Design review of the part built by this model. Coordinates are the model's own, in mm. Face numbers are marked on the shaded views. A direction names the side the tool comes from. Coordinates: 2 decimals unless noted, no trailing zeros. Loops run counter-clockwise (first coordinate to the right, second up) from the corner with the lowest first, then second, coordinate; pieces in that order, holes last. Notation, with made-up numbers: M -33,-13.75 L 1,-13.75 A25 ccw 1,5.25 Z; hole C 66,21 d6. An arc over 180 degrees is marked long. Put each result on its own line as item: value. Start each with the question number.
(1) For probe 1 along Z at (x, y) = (25, -8.5); probe 2 along X at (y, z) = (-26, 50.5); probe 3 along Z at (x, y) = (5, -20.5), list the stretches that pass through material, from the lowest coordinate up. Write a range as [from, to].
(2) Take a section at C-C, the plane y = -27.5. Give the boundary of the cut face in (x, z).
(3) Take a section at D-D, the plane z = 55. Give the boundary of the cut face in (x, y), then the cut area to 3 significant figures.
(4) Clearance check with flat-ended pins moving along their axes: pin 1 (2 mm diameter, centred on y = -11, z = 16, fed in from -X); pin 2 (4 mm diameter, centred on y = -5, z = 16, fed in from -X); pin 3 (10 mm diameter, centred on y = -6, z = 40, fed in from +X). State where each tip first meets the part, or that it passes through.
(5) Take a section at B-B, the plane x = 25.4. Give the boundary of the cut face in (y, z).
(6) The part is to be moulded in two halves that separate along X. For the marked faces 6, 7 and 8, say which applies: +X half, -X half, draft (parallel to the pull), parting line (faces both ways), or undercut.
(7) Take a section at A-A, the plane y = -14. Give the boundary of the cut face in (x, z).
(8) For the marked faces 1, 2, 3, 4 and 5, list the 3-axis set-ups (+Z, -Z, +X, -X, +Y, -Y) from which the entire face can be reached by the end or side of a thin tool; tool diameter is ignored.
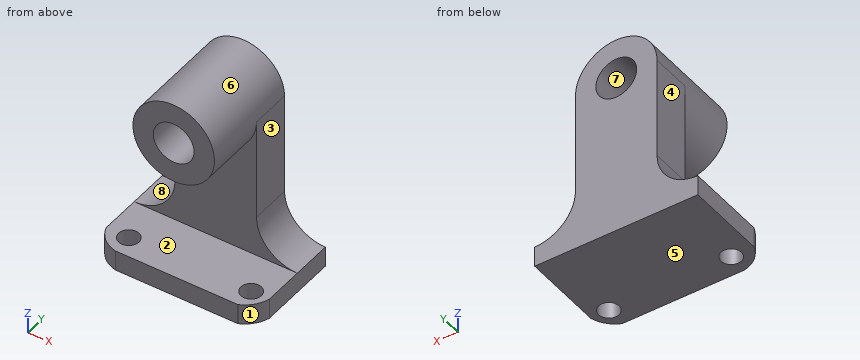
```python
from build123d import *

# Parameters (mm, degrees)
F1_DEPTH  = 31.75
F2_W      = 19.05
F2_H      = 31.75
F3_DEPTH  = 57.15
F5_DEPTH  = 19.05
F7_DEPTH  = 25.4
F8_R      = 6.35
F9_DEPTH  = 31.75
F11_DEPTH = 6.35
F12_R     = 3.175
F13_DEPTH = 6.35
F14_DEPTH = 6.35


with BuildPart() as f1:
    # F0 (on Front) → F1 (new body)
    with BuildSketch(Plane.XZ):
        Polygon((0, 6.35), (0, 0), (50.8, 0), (50.8, 6.35), (50.8, 63.5), (0, 63.5), align=None)
    extrude(amount=F1_DEPTH)

    # F2 (on face) → F3 (cut)
    with BuildSketch(Plane.YZ.offset(50.8)):
        with Locations((-22.225, 22.225)):
            Rectangle(F2_W, F2_H)
    extrude(amount=-F3_DEPTH, mode=Mode.SUBTRACT)

    # F4 (on face) → F5 (cut)
    with BuildSketch(Plane.XZ.offset(31.75)):
        with BuildLine():
            ThreePointArc((25.4, 63.5), (34.3802561211, 59.7802561211), (38.1, 50.8))
            ThreePointArc((38.1, 50.8), (34.3802561211, 41.8197438789), (25.4, 38.1))
            Line((25.4, 38.1), (50.8, 38.1))
            Line((50.8, 38.1), (50.8, 63.5))
            Line((50.8, 63.5), (25.4, 63.5))
        make_face()
        with BuildLine():
            ThreePointArc((25.4, 38.1), (12.7, 50.8), (25.4, 63.5))
            Line((25.4, 63.5), (0, 63.5))
            Line((0, 63.5), (0, 38.1))
            Line((0, 38.1), (25.4, 38.1))
        make_face()
    extrude(amount=-F5_DEPTH, mode=Mode.SUBTRACT)

    # F6 (on face) → F7 (cut)
    with BuildSketch(Plane.XZ.offset(12.7)):
        with BuildLine():
            Line((0, 63.5), (0, 6.35))
            ThreePointArc((0, 6.35), (8.9802561211, 10.0697438789), (12.7, 19.05))
            Line((12.7, 19.05), (12.7, 50.8))
            ThreePointArc((12.7, 50.8), (16.4197438789, 59.7802561211), (25.4, 63.5))
            Line((25.4, 63.5), (0, 63.5))
        make_face()
        with BuildLine():
            ThreePointArc((38.1, 19.05), (41.8197438789, 10.0697438789), (50.8, 6.35))
            Line((50.8, 6.35), (50.8, 63.5))
            Line((50.8, 63.5), (25.4, 63.5))
            ThreePointArc((25.4, 63.5), (34.3802561211, 59.7802561211), (38.1, 50.8))
            Line((38.1, 50.8), (38.1, 19.05))
        make_face()
    extrude(amount=-F7_DEPTH, mode=Mode.SUBTRACT)

    # F8 (on face) → F9 (cut)
    with BuildSketch(Plane.XZ.offset(31.75)):
        with Locations((25.4, 50.8)):
            Circle(F8_R)
    extrude(amount=-F9_DEPTH, mode=Mode.SUBTRACT)

    # F10 (on face) → F11 (cut)
    with BuildSketch(Plane.XY.offset(6.35)):
        with BuildLine():
            Line((0, -25.4), (0, -31.75))
            Line((0, -31.75), (7.2559140616, -31.75))
            ThreePointArc((7.2559140616, -31.75), (2.7651010981, -29.5609540937), (0, -25.4))
        make_face()
        with BuildLine():
            ThreePointArc((50.8, -25.4), (48.8122601511, -29.2045447704), (45.3559140616, -31.75))
            Line((45.3559140616, -31.75), (50.8, -31.75))
            Line((50.8, -31.75), (50.8, -25.4))
        make_face()
    extrude(amount=-F11_DEPTH, mode=Mode.SUBTRACT)

    # F12 (on face) → F13 (cut)
    with BuildSketch(Plane.XY.offset(6.35)):
        with Locations((7.0587542899, -25.4)):
            Circle(F12_R)
        with Locations((45.1587542899, -25.4)):
            Circle(F12_R)
    extrude(amount=-F13_DEPTH, mode=Mode.SUBTRACT)

    # F12 (on face) → F14 (cut)
    with BuildSketch(Plane.XY.offset(6.35)):
        with Locations((7.0587542899, -25.4)):
            Circle(F12_R)
        with Locations((45.1587542899, -25.4)):
            Circle(F12_R)
    extrude(amount=-F14_DEPTH, mode=Mode.SUBTRACT)


solid = f1.part
```
Computed values:
1. probe 1: z = [0, 44.46], [57.14, 63.49]
1. probe 2: x = [12.7, 19.06], [31.74, 38.1]
1. probe 3: z = [0, 6.35]
2. outline: M 1,0 L 4.68,0 L 4.68,6.35 L 1,6.35 Z; M 9.44,0 L 42.78,0 L 42.78,6.35 L 9.44,6.35 Z; C 25.4,50.8 d25.4; M 47.54,0 L 49.98,0 L 49.98,6.35 L 47.54,6.35 Z; hole C 25.4,50.8 d12.7
3. outline: M 13.41,-31.75 L 20.64,-31.75 L 20.64,0 L 13.41,0 Z; M 30.16,-31.75 L 37.39,-31.75 L 37.39,0 L 30.16,0 Z
3. area: 459 mm^2
4. pin 1: stops at x = 12.04
4. pin 2: stops at x = 11.65
4. pin 3: stops at x = 38.1
5. outline: M -31.75,0 L 0,0 L 0,44.45 L -31.75,44.45 L -31.75,38.1 L -12.7,38.1 L -12.7,6.35 L -31.75,6.35 Z; M -31.75,57.15 L 0,57.15 L 0,63.5 L -31.75,63.5 Z
6. face 6: parting line
6. face 7: undercut
6. face 8: -X half
7. outline: M 0,0 L 50.8,0 L 50.8,6.35 L 0,6.35 Z; C 25.4,50.8 d25.4; hole C 25.4,50.8 d12.7
8. face 1: +Z, -Z, +X, -Y
8. face 2: +X, -X, -Y
8. face 3: +Z, +X, +Y, -Y
8. face 4: +Z, -X, +Y, -Y
8. face 5: -Z, +X, -X, +Y, -Y
